The listing builds one solid part. Answer for the finished solid, in the listing's coordinates (mm). Face numbers are marked on the shaded views. A direction names the side the tool comes from. Round coordinates to 2 decimals unless told otherwise and drop trailing zeros. Write each loop counter-clockwise with the first axis right and the second up, starting at its lowest first coordinate (ties: lowest second). Pieces come first, ordered by that corner, then holes.
Item 1: Find section A-A on y = -9.5. Give the vertices of the cut face in (x, z), then the cut area to 3 significant figures.
Item 2: A tool of negligible diameter and unlimited length cuts with its end or side. For the marked faces 1, 2 and 3, from which of +Z, -Z, +X, -X, +Y, -Y can it reach the whole face along a straight path? Write none if from no direction.
Item 3: Find section B-B on z = -12.5. Give the vertices of the cut face in (x, y), then the cut area to 4 significant figures.
Item 4: Find the intervals of material crossed by probe 1 along X at (y, z) = (-5, 12.5); probe 2 along Y at (x, z) = (19.5, 0); probe 3 along Z at (x, y) = (23, -15.75) (3 decimals), in increasing order.
Item 5: For a pull along Z with two mould halves and no side action, classify the marked faces 4, 5, 6 and 7 as +Z half, -Z half, draft (parallel to the pull), parting line (faces both ways), or undercut.
Item 6: Find section D-D on z = 0. Give the vertices of the cut face in (x, y), then the cut area to 3 significant figures.
Item 7: Each of these flat-tipped pins is pushed along its axis until it touches: pin 1 (8 mm diameter, centred on y = -10, z = 3, fed in from +X) (3 decimals); pin 2 (2 mm diameter, centred on x = 10.5, y = -6.5, fed in from +Z); pin 3 (6.5 mm diameter, centred on x = 15, z = 12, fed in from -Y); pin 4 (10 mm diameter, centred on x = 21.5, z = 12, fed in from +Y). Where does it stop, or does it pass through?
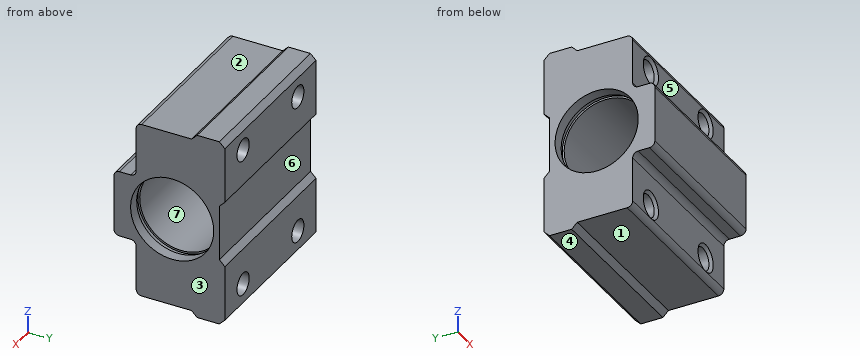
Autodesk Inventor part; units mm, degrees
ref_plane "Płaszczyzna konstrukcyjna2" through (2, 0, 0) normal (-1, 0, 0) x (0, 0, 1)
ref_plane "Płaszczyzna konstrukcyjna3" through (15, 0, 0) normal (-1, 0, 0) x (0, 0, 1)
ref_plane "YZ Plane" through (0, 0, 0) normal (1, 0, 0) x (0, 1, 0)
sketch "Szkic1" plane through (0, 0, 0) normal (1, 0, 0) x (0, 1, 0)
  line L0 (0, 17) -> (-6, 17)
  line L1 (-6, 17) -> (-6, 16)
  line L2 (-6, 16) -> (-16, 16)
  line L3 (-16, 16) -> (-16, 6)
  line L4 (-16, 6) -> (-20, 6)
  line L5 (-20, 6) -> (-20, 0)
  line L6 (0, 17) -> (0, 5)
  line L7 (0, 5) -> (-1, 5)
  line L8 (-1, 5) -> (-1, 0)
  line L9 (-1, 0) -> (-20, 0) construction
  line L10 (0, -17) -> (-6, -17)
  line L11 (-6, -17) -> (-6, -16)
  line L12 (-6, -16) -> (-16, -16)
  line L13 (-16, -16) -> (-16, -6)
  line L14 (-16, -6) -> (-20, -6)
  line L15 (-20, -6) -> (-20, 0)
  line L16 (0, -17) -> (0, -5)
  line L17 (0, -5) -> (-1, -5)
  line L18 (-1, -5) -> (-1, 0)
  point P0 (0, 0)
  dimension "d0" = 17
  dimension "d1" = 6
  dimension "d2" = 1
  dimension "d3" = 10
  dimension "d4" = 10
  dimension "d5" = 4
  dimension "d40" = 12
  dimension "d41" = 1
  dimension "d43" = 6
extrude "Wyciągnięcie proste1" add sketch "Szkic1" along normal blind 30
ref_plane "Płaszczyzna konstrukcyjna2" through (2, 0, 0) normal (-1, 0, 0) x (0, 0, 1)
ref_plane "Płaszczyzna konstrukcyjna3" through (15, 0, 0) normal (-1, 0, 0) x (0, 0, 1)
sketch "Szkic7" plane through (0, 0, 0) normal (-1, 0, 0) x (0, 0, 1)
  line L0 (6, -20) -> (-6, -20)
  point P0 (0, 0)
  point P1 (0, -9.5)
  dimension "d44" = 10.5
hole "Otwór3" at (0, -9.5, 0) direction (1, 0, 0) diameter 15 end through all
sketch "Szkic8" plane through (2, 0, 0) normal (-1, 0, 0) x (0, 0, 1)
  circle A0 centre (0, -9.5) radius 7.5
  circle A1 centre (0, -9.5) radius 7.85
  point P0 (0, 0)
  dimension "d52" = 15.7
extrude "Wyciągnięcie proste4" cut sketch "Szkic8" against normal blind 1
mirror "Odbij2" about plane through (15, 0, 0) normal (-1, 0, 0) of "Wyciągnięcie proste4"
sketch "Szkic9" plane through (0, 0, 17) normal (0, 1, 0) x (1, 0, 0)
  line L0 (0, 0) -> (30, 0)
  line L1 (30, 12) -> (30, 0)
  point P0 (0, 17)
  point P1 (24, 29.5)
  point P2 (24, 4.5)
  point P3 (6, 4.5)
  point P4 (6, 29.5)
  dimension "d55" = 18
  dimension "d56" = 25
  dimension "d57" = 4.5
  dimension "d58" = 6
chamfer "Faza2" distance 1 angle 45 6 edges at (15, 0, 5) (15, 0, -5) (15, 0, 17) (15, 0, -17) (15, -6, -17) (15, -6, 17)
fillet "Zaokrąglenie2" radius 1 6 edges at (15, -16, 16) (15, -20, 6) (15, -20, -6) (15, -16, -16) (15, -16, 6) (15, -16, -6)
hole "Otwór5" at (24, 0, -12.5) at (24, 0, 12.5) at (6, 0, 12.5) at (6, 0, -12.5) direction (0, -1, 0) diameter 4 end through all
chamfer "Faza3" distance 0.5 angle 45 4 edges at (24, -16, 10.5) (6, -16, 10.5) (24, -16, -14.5) (6, -16, -14.5)
properties part number "16_obudowa łożyska"
Check values:
1. outline: (0, -16) - (30, -16) - (30, -7.5) - (28, -7.5) - (28, -7.85) - (27, -7.85) - (27, -7.5) - (3, -7.5) - (3, -7.85) - (2, -7.85) - (2, -7.5) - (0, -7.5) - close; (0, 7.5) - (2, 7.5) - (2, 7.85) - (3, 7.85) - (3, 7.5) - (27, 7.5) - (27, 7.85) - (28, 7.85) - (28, 7.5) - (30, 7.5) - (30, 16) - (0, 16) - close; hole circle Ø4 at (6, -12.5); hole circle Ø4 at (6, 12.5); hole circle Ø4 at (24, -12.5); hole circle Ø4 at (24, 12.5)
1. area: 458 mm2
2. face 1: -Z, +X, -X, -Y
2. face 2: +Z, +X, -X, -Y
2. face 3: +Z, -Z, +X, +Y, -Y
3. outline: (0, -16) - (3.5, -16) - (4, -15.5) - (4, 0) - (0, 0) - close; (8, -15.5) - (8.5, -16) - (21.5, -16) - (22, -15.5) - (22, 0) - (8, 0) - close; (26, -15.5) - (26.5, -16) - (30, -16) - (30, 0) - (26, 0) - close
3. area: 351.5 mm2
4. probe 1: x = 0 to 4, 8 to 22, 26 to 30
4. probe 2: y = -20 to -17, -2 to -1
4. probe 3: z = -15.661 to -14.515, -10.485 to -4.146, 4.146 to 10.485, 14.515 to 15.661
5. face 4: -Z half
5. face 5: draft
5. face 6: undercut
5. face 7: undercut
6. outline: (0, -20) - (30, -20) - (30, -17) - (28, -17) - (28, -17.35) - (27, -17.35) - (27, -17) - (3, -17) - (3, -17.35) - (2, -17.35) - (2, -17) - (0, -17) - close; (0, -2) - (2, -2) - (2, -1.65) - (3, -1.65) - (3, -2) - (27, -2) - (27, -1.65) - (28, -1.65) - (28, -2) - (30, -2) - (30, -1) - (0, -1) - close
6. area: 119 mm2
7. pin 1: passes through
7. pin 2: stops at z = 16.5
7. pin 3: stops at y = -16
7. pin 4: stops at y = 0
